Verification items for the finished model (mm, model axes). Coordinates: 2 decimals unless noted, no trailing zeros. Order: outer loops, then holes, each group sorted by start corner. A loop starts at its lowest first (then second) coordinate and runs counter-clockwise, first axis right, second up. Notation, with made-up numbers: (-7.75, 36.5) -> (19.25, 36.5) arc R20 ccw to (19.25, 69.5) -> close; hole circle Ø1 at (-27.75, 1.5). An arc over 180 degrees is marked (long way). Write item = value, one per line. Start each with the question number.
1. Cross-section at C-C on x = 22.5. Record the cut outline in (y, z), plus the area to 3 significant figures.
2. Cross-section at A-A on x = 99. Record the cut outline in (y, z), plus the area to 3 significant figures.
3. Thickness scan on line 1 along Y through (x, z) = (15, 1.95); line 2 along X through (y, z) = (-82.5, 1.2); line 3 along X through (y, z) = (-177, 1.7). Record the ranges inside material, lowest first. Write a range as from..to.
4. Go/stop test with flat-tipped pins: P1, Ø1.5, axis at y = -88, z = 2, coming from the +X side; P2, Ø0.9, axis at y = -189, z = 2, coming from the -X side; P3, Ø1.5, axis at x = 54.5, z = 1.5, coming from the -Y side. Record where each tip stops, or that it passes through.
5. Cross-section at D-D on y = -6.5. Record the cut outline in (x, z).
6. Cross-section at B-B on y = -120. Record the cut outline in (x, z).
from build123d import *

# Parameters (mm, degrees)
F0_W     = 3.5
F0_H     = 40
F0_W_2   = 5
F1_DEPTH = 3
F2_R     = 5
F3_R     = 4.99999
F4_R     = 4.99999


# Not quite as in the source:
# - a fillet or chamfer is up to 0.001 mm smaller than in the source, because OpenCascade refuses the exact size


with BuildPart() as f1:
    # F0 (on Top) → F1 (new body)
    with BuildSketch(Plane.XY):
        Polygon((129.5, -200), (199, -200), (199, -157), (202, -157), (202, -117), (199, -117), (199, -77), (202, -77), (202, -37), (199, -37), (199, 6), (129.5, 6), (129.5, -37), (126, -37), (126, 6), (56.5, 6), (56.5, -37), (53, -37), (53, 6), (3, 6), (3, -37), (0, -37), (0, -77), (3, -77), (3, -117), (0, -117), (0, -157), (3, -157), (3, -200), (53, -200), (53, -157), (56.5, -157), (56.5, -200), (126, -200), (126, -157), (129.5, -157), align=None)
        Polygon((33, -134.75), (33, -137), (33, -139.25), (13, -139.25), (13, -134.75), align=None, mode=Mode.SUBTRACT)
        with Locations((54.75, -97)):
            Rectangle(F0_W, F0_H, mode=Mode.SUBTRACT)
        Polygon((61.5, -195), (61.5, -97), (61.5, 0), (121.5, 0), (121.5, -50), (111.5, -50), (111.5, -145), (121.5, -145), (121.5, -195), align=None, mode=Mode.SUBTRACT)
        with Locations((119, -97)):
            Rectangle(F0_W_2, F0_H, mode=Mode.SUBTRACT)
        with Locations((127.75, -97)):
            Rectangle(F0_W, F0_H, mode=Mode.SUBTRACT)
        Polygon((33, -54.75), (33, -57), (33, -59.25), (13, -59.25), (13, -54.75), align=None, mode=Mode.SUBTRACT)
    extrude(amount=F1_DEPTH)

    # F2
    f2_edges = [f1.edges().sort_by_distance(p)[0] for p in [
        (121.5, -50, 1.5),
    ]]
    fillet(f2_edges, radius=F2_R)

    # F3 (radius 5 in the source; OpenCascade refuses exactly that, so slightly less here)
    f3_edges = [f1.edges().sort_by_distance(p)[0] for p in [
        (111.5, -50, 1.5),
    ]]
    fillet(f3_edges, radius=F3_R)

    # F4 (radius 5 in the source; OpenCascade refuses exactly that, so slightly less here)
    f4_edges = [f1.edges().sort_by_distance(p)[0] for p in [
        (121.5, -145, 1.5),
        (111.5, -145, 1.5),
    ]]
    fillet(f4_edges, radius=F4_R)


solid = f1.part
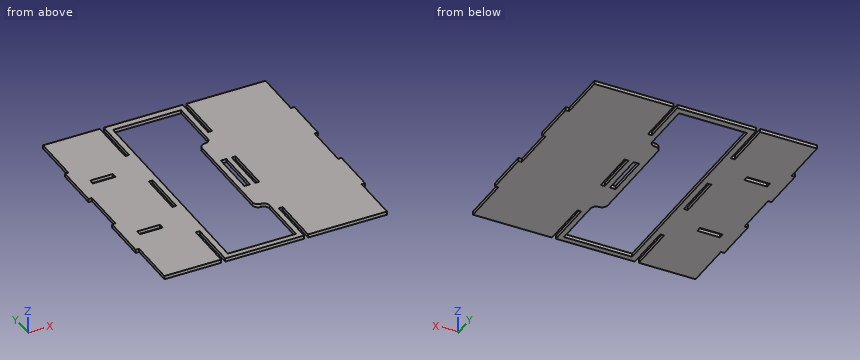
Worked out:
q1.outline = (-200, 0) -> (-139.25, 0) -> (-139.25, 3) -> (-200, 3) -> close; (-134.75, 0) -> (-59.25, 0) -> (-59.25, 3) -> (-134.75, 3) -> close; (-54.75, 0) -> (6, 0) -> (6, 3) -> (-54.75, 3) -> close
q1.area = 591 mm²
q2.outline = (-200, 0) -> (-195, 0) -> (-195, 3) -> (-200, 3) -> close; (0, 0) -> (6, 0) -> (6, 3) -> (0, 3) -> close
q2.area = 33.0 mm²
q3.line_1 = -200..-139.25, -134.75..-59.25, -54.75..6
q3.line_2 = 3..53, 56.5..61.5, 111.5..116.5, 121.5..126, 129.5..199
q3.line_3 = 3..53, 56.5..61.5, 121.5..126, 129.5..199
q4.P1 = 199
q4.P2 = 3
q4.P3 = -157
q5.outline = (3, 0) -> (53, 0) -> (53, 3) -> (3, 3) -> close; (56.5, 0) -> (61.5, 0) -> (61.5, 3) -> (56.5, 3) -> close; (121.5, 0) -> (126, 0) -> (126, 3) -> (121.5, 3) -> close; (129.5, 0) -> (199, 0) -> (199, 3) -> (129.5, 3) -> close
q6.outline = (0, 0) -> (61.5, 0) -> (61.5, 3) -> (0, 3) -> close; (111.5, 0) -> (202, 0) -> (202, 3) -> (111.5, 3) -> close
